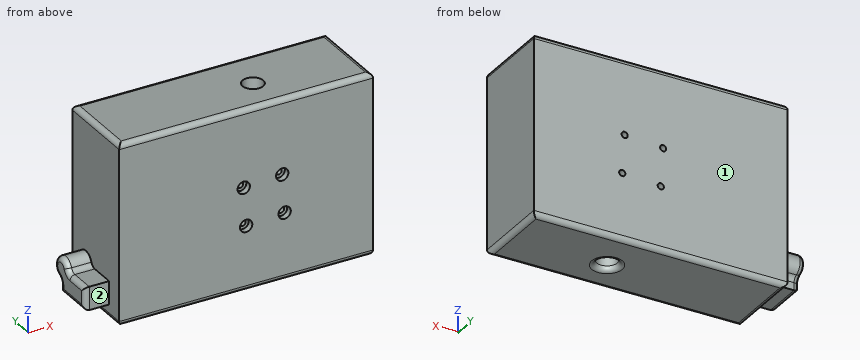
from build123d import *

# Parameters (mm, degrees)
F0_W            = 260.7417907566
F0_H            = 185.2982528508
F1_DEPTH        = 83.312
F2_R            = 5.08
F3_R            = 10.6560791483
F4_DEPTH        = 185.2982528508
F6_DEPTH        = 25.4
F7_R            = 5.08
F9_D            = 6.35
F9_CBORE_D      = 12.7
F9_CBORE_DEPTH  = 6.35
F9_COPIES_COUNT = 4


# Not quite as in the source:
# - a pattern or mirror of a feature is missing from the dataset's text; its kind, count and spacing are read off the source's solid


with BuildPart() as f1:
    # F0 (on Front) → F1 (new body)
    with BuildSketch(Plane.XZ):
        with Locations((-18.5430413112, 5.6122671813)):
            Rectangle(F0_W, F0_H)
    extrude(amount=F1_DEPTH)

    # F2
    f2_edges = [f1.edges().sort_by_distance(p)[0] for p in [
        (-148.913937, -41.656, 98.261394),
        (-18.543041, -83.312, 98.261394),
        (111.827854, -41.656, 98.261394),
        (-18.543041, 0, 98.261394),
    ]]
    fillet(f2_edges, radius=F2_R)

    # F3 (on face) → F4 (cut, through all)
    with BuildSketch(Plane.XY.offset(98.2613936067)):
        with Locations((10.0774681196, -45.8871424198)):
            Circle(F3_R)
    extrude(amount=-F4_DEPTH, mode=Mode.SUBTRACT)

    # F5 (on face) → F6 (join)
    with BuildSketch(Plane(origin=(-148.9139366895, 0, 0), x_dir=(0, -1, 0), z_dir=(-1, 0, 0))):
        with BuildLine():
            ThreePointArc((39.8253589774, -49.4220387191), (36.2562578791, -48.3240875907), (33.9213925534, -45.4099181994))
            ThreePointArc((33.9213925534, -45.4099181994), (16.0837066862, -41.7163656596), (19.777259226, -59.5540515267))
            ThreePointArc((19.777259226, -59.5540515267), (22.6914286173, -61.8889168524), (23.7893797457, -65.4580179507))
            Line((23.7893797457, -65.4580179507), (23.7893797457, -73.2655222528))
            Line((23.7893797457, -73.2655222528), (65.4315222055, -73.2655222528))
            Line((65.4315222055, -73.2655222528), (65.4315222055, -49.4220387191))
            Line((65.4315222055, -49.4220387191), (39.8253589774, -49.4220387191))
        make_face()
    extrude(amount=F6_DEPTH)

    # F7
    f7_edges = [f1.edges().sort_by_distance(p)[0] for p in [
        (-174.313937, -65.431522, -61.34378),
        (-174.313937, -52.628441, -49.422039),
        (-174.313937, -36.256258, -48.324088),
        (-174.313937, -16.083707, -41.716366),
        (-174.313937, -22.691429, -61.888917),
        (-174.313937, -23.78938, -69.36177),
        (-174.313937, -44.610451, -73.265522),
        (-148.913937, -41.656, -87.036859),
        (-18.543041, 0, -87.036859),
        (-18.543041, -83.312, -87.036859),
        (111.827854, -41.656, -87.036859),
        (-0.578611, -45.887142, -87.036859),
    ]]
    fillet(f7_edges, radius=F7_R)

    # F9 (through all)
    with Locations(Plane.XZ.offset(83.312)):
        with Locations((-18.5430413112, -21.0058055818)):
            f9 = CounterBoreHole(F9_D / 2, F9_CBORE_D / 2, F9_CBORE_DEPTH)

    # F9_copies: F9 ×4 about axis
    f9_copies_axis = Axis((0, 0, 0), (0, 1, 0))
    for i in range(1, F9_COPIES_COUNT):
        add(f9.rotate(f9_copies_axis, i * 360 / F9_COPIES_COUNT), mode=Mode.SUBTRACT)


solid = f1.part
Geometry check sheet. Reference: the model listing, model coordinates, mm. Face numbers are marked on the shaded views. A direction names the side the tool comes from. Round coordinates to 2 decimals unless told otherwise and drop trailing zeros. Loops run counter-clockwise (first coordinate to the right, second up) from the corner with the lowest first, then second, coordinate; pieces in that order, holes last. Notation, with made-up numbers: (49.5, 26) - (77.5, 26) arc R30 cw to (77.5, 63) - close; hole circle Ø10 at (82.5, 34). An arc over 180 degrees is marked (long way). One line per question, with ' | ' between items. Start each with the question number.
1. Cross-section at A-A on z = 59.5. Record the cut outline in (x, y).
2. Tool access check on the marked faces 1 and 2. Record the directions out of +Z, -Z, +X, -X, +Y, -Y that give a thin tool (end or side, any length) a straight path to the whole face; none if there is none.
3. Cross-section at B-B on y = -51.5. State how many separate pieces and enclosed holes the cut face has, then the cut area to 3 significant figures.
4. Scan lines: line 1 (Z direction, x = -19, y = -55); line 2 (X direction, y = -78, z = 78); line 3 (X direction, y = -41, z = -17.5). Record each from-to range of solid material in increasing order. Write a range as [from, to].
5. Depth check by flat-ended pin: pin 1 (1 mm diameter, centred on y = -12.5, z = -26.5, fed in from -X); pin 2 (7.5 mm diameter, centred on x = -18.54, z = -21.01, fed in from -Y); pin 3 (16.5 mm diameter, centred on x = -157.5, z = -61, fed in from -Y); pin 4 (5 mm diameter, centred on x = -21.01, z = 18.54, fed in from +Y). Enter the tip coordinate at first touch or a pass-through.
Taken from the geometry:
1) outline: (-148.91, -83.31) - (111.83, -83.31) - (111.83, 0) - (-148.91, 0) - close; hole circle Ø21.31 at (10.08, -45.89)
2) face 1: +Z, -Z, +X, -X, +Y | face 2: +Z, -Z, -X, -Y
3) separate pieces: 2 | enclosed holes: 2 | area: 45,400 mm²
4) line 1: [-87.04, -24.15], [-17.86, 16.08], [21, 98.26] | line 2: [-148.91, 111.83] | line 3: [-148.91, 0.61], [24, 111.83]
5) pin 1: x = -148.91 | pin 2: y = -76.96 | pin 3: y = -65.43 | pin 4: through
